Check sheet for the modelled part. Datum: model origin and axes. Units: mm. Face numbers are marked on the shaded views. A direction names the side the tool comes from. Give positions to 0.01 mm unless a question says otherwise; leave off trailing zeros. Write each loop counter-clockwise with the first axis right and the second up, starting at its lowest first coordinate (ties: lowest second). Pieces come first, ordered by that corner, then holes. Notation, with made-up numbers: (80.5, 10.25) -> (101.5, 10.25) arc R31 ccw to (101.5, 36.25) -> close; hole circle Ø11 at (37.25, 39). An arc over 180 degrees is marked (long way). Use a Markdown table: item, result. Add a question column.
1. Scan lines: probe 1 along X at (y, z) = (15, 1.05); probe 2 along X at (y, z) = (23.5, 1.1); probe 3 along Y at (x, z) = (15, 1.1). Record each from-to range of solid material in increasing order. Write a range as [from, to].
2. Cross-section at B-B (y = 15). Enter the section's corners in (x, z), then the cut area to 3 significant figures.
3. Set-up check for the marked faces 1 and 2: record each of +Z, -Z, +X, -X, +Y, -Y from which the full face is reachable in a straight line by a thin tool's end or side.
4. Gauge pin test, flat ends, axial feed: P1, Ø2, axis at x = 25, z = 20, coming from the -Y side; P2, Ø10, axis at x = 6.5, z = 17.5, coming from the -Y side; P3, Ø3, axis at x = 5.5, y = 36, coming from the -Z side. Record the tip position at first contact, or that the pin passes through.
5. Cross-section at A-A (y = 23.5). Enter the section's corners in (x, z).
6. Cross-section at D-D (x = 21.5). Enter the section's corners in (y, z), then the cut area to 3 significant figures.
7. Cross-section at C-C (x = 6.5). Enter the section's corners in (y, z).
Autodesk Inventor part; units mm, degrees
ref_plane "YZ Plane" through (0, 0, 0) normal (1, 0, 0) x (0, 1, 0)
ref_plane "XZ Plane" through (0, 0, 0) normal (0, 1, 0) x (-1, 0, 0)
ref_plane "XY Plane" through (0, 0, 0) normal (0, 0, 1) x (1, 0, 0)
sketch "スケッチ2" plane through (0, 0, 0) normal (0, 0, 1) x (1, 0, 0)
  line L0 (0, 0) -> (30, 0)
  line L1 (30, 0) -> (30, 30)
  line L2 (30, 30) -> (0, 30)
  line L3 (0, 30) -> (0, 0)
  dimension "d0" = 30
  dimension "d1" = 30
extrude "プレート1" add sketch "スケッチ2" along normal blind 1.5
sketch "スケッチ5" plane through (0, 28.9393, 1.0607) normal (0, 0.7071068, -0.7071068) x (-1, 0, 0)
  line L0 (-30, 0) -> (0, 0)
  line L1 (0, 0) -> (0, 40)
  line L2 (0, 40) -> (-30, 40)
  line L3 (-30, 40) -> (-30, 0)
edge flange "フランジ1" height 40 angle 45 thickness 1.5 bend radius 1.5 thickness toward (0, 0.7071068, -0.7071068) relief tear relief width 1.5 relief depth 0.75 edges at (15, 30, 1.5) wall of the first edge with corners at (30, 28.9393, 1.0607) (0, 28.9393, 1.0607) (0, 57.2236, 29.3449) (30, 57.2236, 29.3449)
bend "曲げ1"
corner "コーナー1"
sketch "スケッチ6" plane through (0, 0, 1.5) normal (0, 0, 1) x (1, 0, 0)
  line L0 (30, 0) -> (0, 0)
  line L1 (15, 0) -> (15, 28.7574) construction
  line L2 (30, 28.7574) -> (0, 28.7574)
  line L3 (0, 0) -> (0, 28.7574)
  line L4 (0, 15) -> (30, 15) construction
  point P0 (15, 15)
  dimension "d34" = 15
hole "穴3" at (15, 15, 1.5) direction (0, 0, -1) diameter 10 end through all
sketch "スケッチ7" plane through (0, 0, 1.5) normal (0, 0, 1) x (1, 0, 0)
  circle A0 centre (15, 15) radius 5
  line L0 (30, 28.7574) -> (0, 28.7574)
  line L1 (0, 0) -> (0, 28.7574)
  line L2 (30, 0) -> (0, 0)
  line L3 (30, 28.7574) -> (30, 0)
  line L4 (15, 15) -> (30, 15) construction
  line L5 (30, 0) -> (30, 28.7574)
  line L6 (15, 15) -> (15, 30) construction
  line L7 (15, 15) -> (0, 15) construction
  line L8 (15, 15) -> (15, 0) construction
  point P0 (23.5, 15)
  point P1 (15, 23.5)
  point P2 (6.5, 15)
  point P3 (15, 6.5)
  dimension "d42" = 8.5
  dimension "d45" = 360
hole "穴4" at (23.5, 15, 1.5) at (15, 23.5, 1.5) at (6.5, 15, 1.5) at (15, 6.5, 1.5) direction (0, 0, -1) diameter 2.8 end through all
sketch "スケッチ8" plane through (0, 57.2236, 29.3449) normal (0, -0.7071068, 0.7071068) x (1, 0, 0)
  line L0 (30, 0) -> (0, 0)
  line L1 (15, 0) -> (15, -38.7574) construction
  line L2 (0, -38.7574) -> (30, -38.7574)
  line L3 (0, -38.7574) -> (0, 0)
  line L4 (0, -15) -> (29.8306, -15) construction
  point P0 (0, -61.2132)
  point P1 (14.9153, -15)
  dimension "d54" = 15
hole "穴5" at (14.9153, 46.617, 18.7383) direction (0, 0.7071068, -0.7071068) diameter 20 end through all
equation "\"d23\" = Thickness"
equation "\"d24\" = BendReliefWidth"
equation "\"d25\" = BendReliefDepth"
equation "\"d26\" = MinimumRemnant"
equation "\"d27\" = TransitionRadius"
equation "\"d30\" = BendRadius"
equation "\"d31\" = CornerReliefSize"
equation "\"d32\" = GapSize"
equation "\"d33\" = JacobiRadiusSize"
equation "\"BendRadius\" = Thickness"
equation "\"BendReliefWidth\" = Thickness"
equation "\"BendReliefDepth\" = 0.5 * Thickness"
equation "\"CornerReliefSize\" = 4 * Thickness"
equation "\"MinimumRemnant\" = 2 * Thickness"
equation "\"TransitionRadius\" = BendRadius"
equation "\"JacobiRadiusSize\" = BendRadius"
equation "\"GapSize\" = Thickness"
properties part number "head"
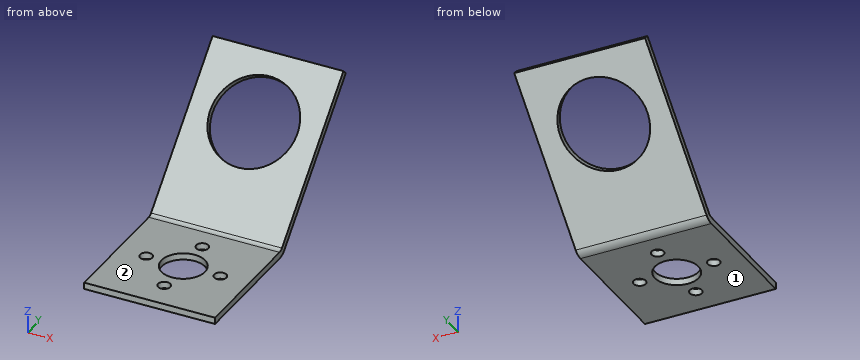
Worked answers:
| question | item | result |
|---|---|---|
| 1 | probe 1 | x = [0, 5.1], [7.9, 10], [20, 22.1], [24.9, 30] |
| 1 | probe 2 | x = [0, 13.6], [16.4, 30] |
| 1 | probe 3 | y = [0, 5.1], [7.9, 10], [20, 22.1], [24.9, 31.1] |
| 2 | outline | (0, 0) -> (5.1, 0) -> (5.1, 1.5) -> (0, 1.5) -> close; (7.9, 0) -> (10, 0) -> (10, 1.5) -> (7.9, 1.5) -> close; (20, 0) -> (22.1, 0) -> (22.1, 1.5) -> (20, 1.5) -> close; (24.9, 0) -> (30, 0) -> (30, 1.5) -> (24.9, 1.5) -> close |
| 2 | area | 21.6 mm² |
| 3 | face 1 | -Z, +X, -X, +Y, -Y |
| 3 | face 2 | +Z, +X, -X, -Y |
| 4 | P1 | stops at y = 46.88 |
| 4 | P2 | stops at y = 40.38 |
| 4 | P3 | stops at z = 4.5 |
| 5 | outline | (0, 0) -> (13.6, 0) -> (13.6, 1.5) -> (0, 1.5) -> close; (16.4, 0) -> (30, 0) -> (30, 1.5) -> (16.4, 1.5) -> close |
| 6 | outline | (0, 0) -> (28.76, 0) arc R3 ccw to (30.88, 0.88) -> (42.36, 12.36) -> (41.3, 13.42) -> (29.82, 1.94) arc R1.5 cw to (28.76, 1.5) -> (0, 1.5) -> close; (51.94, 24.06) -> (53, 23) -> (58.28, 28.28) -> (57.22, 29.34) -> close |
| 6 | area | 81.3 mm² |
| 7 | outline | (0, 0) -> (13.6, 0) -> (13.6, 1.5) -> (0, 1.5) -> close; (16.4, 0) -> (28.76, 0) arc R3 ccw to (30.88, 0.88) -> (43.86, 13.86) -> (42.8, 14.92) -> (29.82, 1.94) arc R1.5 cw to (28.76, 1.5) -> (16.4, 1.5) -> close; (50.44, 22.56) -> (51.5, 21.5) -> (58.28, 28.28) -> (57.22, 29.34) -> close |
